from build123d import *

# Parameters (mm, degrees)
SKETCH_1_W               = 150
SKETCH_1_H               = 150
EXTRUDE_1_DEPTH          = 6
CHAMFER_1_SIZE           = 5
SKETCH_2_R               = 1.5
CUT_EXTRUDE_1_DEPTH      = 10
SKETCH_3_R               = 2.85
CUT_EXTRUDE_2_DEPTH      = 3.2
MIRROR_2_COPY_1_SKETCH_R = 2.85
MIRROR_2_COPY_1_DEPTH    = 3.2
HOLE_WIZARD_M3_1_D       = 2.5
HOLE_WIZARD_M3_1_DEPTH   = 7.5
HOLE_WIZARD_M3_1_TIP     = 0.751075774
HOLE_WIZARD_M3_2_D       = 2.5
HOLE_WIZARD_M3_2_DEPTH   = 7.5
HOLE_WIZARD_M3_2_TIP     = 0.751075774


with BuildPart() as part:
    # 草图1 → 凸台-拉伸1 (new body)
    with BuildSketch(Plane.XY):
        Rectangle(SKETCH_1_W, SKETCH_1_H)
    extrude(amount=EXTRUDE_1_DEPTH)

    # 倒角1
    chamfer_1_edges = [part.edges().sort_by_distance(p)[0] for p in [
        (-75, 75, 3),
        (75, 75, 3),
        (75, -75, 3),
        (-75, -75, 3),
    ]]
    chamfer(chamfer_1_edges, length=CHAMFER_1_SIZE)

    # 草图2 → 切除-拉伸1 (cut)
    with BuildSketch(Plane.XY.offset(6)):
        with Locations((64, 71)):
            Circle(SKETCH_2_R)
        with Locations((71, 64)):
            Circle(SKETCH_2_R)
        with Locations((-71, 64)):
            Circle(SKETCH_2_R)
        with Locations((-64, 71)):
            Circle(SKETCH_2_R)
    cut_extrude_1 = extrude(amount=-CUT_EXTRUDE_1_DEPTH, mode=Mode.SUBTRACT)

    # 草图3 → 切除-拉伸2 (cut)
    with BuildSketch(Plane(origin=(0, 0, 0), x_dir=(-1, 0, 0), z_dir=(0, 0, -1))):
        with Locations((64, 71)):
            Circle(SKETCH_3_R)
        with Locations((71, 64)):
            Circle(SKETCH_3_R)
    cut_extrude_2 = extrude(amount=-CUT_EXTRUDE_2_DEPTH, mode=Mode.SUBTRACT)

    # 镜向1: 切除-拉伸2 across plane
    add(cut_extrude_2.mirror(Plane(origin=(0, 0, 0), x_dir=(0, 0, 1), z_dir=(1, 0, 0))), mode=Mode.SUBTRACT)

    # 镜向2: 切除-拉伸1, 切除-拉伸2 across plane
    add(cut_extrude_1.mirror(Plane.ZX), mode=Mode.SUBTRACT)
    add(cut_extrude_2.mirror(Plane.ZX), mode=Mode.SUBTRACT)

    # 镜向2 copy 1 sketch → 镜向2 copy 1 (cut)
    with BuildSketch(Plane(origin=(0, 0, 0), x_dir=(1, 0, 0), z_dir=(0, 0, -1))):
        with Locations((64, 71)):
            Circle(MIRROR_2_COPY_1_SKETCH_R)
        with Locations((71, 64)):
            Circle(MIRROR_2_COPY_1_SKETCH_R)
    extrude(amount=-MIRROR_2_COPY_1_DEPTH, mode=Mode.SUBTRACT)

    # M3 螺纹孔1
    with Locations(Plane.XY.offset(6)):
        with Locations((-5.5, -3.5), (5.5, -3.5)):
            Hole(HOLE_WIZARD_M3_1_D / 2, depth=HOLE_WIZARD_M3_1_DEPTH)
            with Locations((0, 0, -(HOLE_WIZARD_M3_1_DEPTH + HOLE_WIZARD_M3_1_TIP / 2))):  # 118° drill point
                Cone(0, HOLE_WIZARD_M3_1_D / 2, HOLE_WIZARD_M3_1_TIP, mode=Mode.SUBTRACT)

    # M3 螺纹孔2
    with Locations(Plane.XY.offset(6)):
        with Locations((-28, 47), (-28, 32)):
            Hole(HOLE_WIZARD_M3_2_D / 2, depth=HOLE_WIZARD_M3_2_DEPTH)
            with Locations((0, 0, -(HOLE_WIZARD_M3_2_DEPTH + HOLE_WIZARD_M3_2_TIP / 2))):  # 118° drill point
                Cone(0, HOLE_WIZARD_M3_2_D / 2, HOLE_WIZARD_M3_2_TIP, mode=Mode.SUBTRACT)


solid = part.part
Could you check a few things on this model? Use its own coordinates, in mm. A direction names the side the tool comes from. Coordinates: 2 decimals unless noted, no trailing zeros. Write item = value, one per line.
1) For faces 4 (the cylindrical face through (66.718, 71.856, 1.578)), 5 (the flat face through (72, 73, 3)), which set-ups out of +Z, -Z, +X, -X, +Y, -Y let a thin tool reach every point of the face, with its end or its side?
Result set:
face_4 = -Z
face_5 = +Z, -Z, +X, +Y
2) We'd pull the mould along Y, two halves only. Please class faces 1 (the flat face through (-75, -1, 3)), 2 (the flat face through (65.2, 69.8, 3.2)), 3 (the flat face through (-72, -73, 3)): +Y half, -Y half, draft (parallel to the pull), parting line (faces both ways), or undercut.
Result set:
face_1 = draft
face_2 = undercut
face_3 = -Y half
3) Will these pins go through, and if not, where does the flat tip stop? pin 1 Ø1.8 at (x, y) = (-71, 64) entering from +Z; pin 2 Ø1.7 at (x, y) = (-64, -70) entering from -Z.
Result set:
pin_1 = through
pin_2 = 3.2
4) Please list where these lines run through material, in increasing order: line 1 (Y direction, x = -64, z = 2.1); line 2 (Y direction, x = 71, z = 5.1). Write a range as [from, to].
Result set:
line_1 = [-75, -73.85], [-68.15, 68.15], [73.85, 75]
line_2 = [-74, -65.5], [-62.5, 62.5], [65.5, 74]
